```python
from build123d import *

# Parameters (mm, degrees)
CYLINDER068_R     = 71
CYLINDER068_DEPTH = 2
CYLINDER069_R     = 71
CYLINDER069_DEPTH = 2


with BuildPart() as cylinder:
    # Cylinder068 → Cylinder068 (new body)
    with BuildSketch(Plane(origin=(105, 148, 35), x_dir=(1, 0, 0), z_dir=(0, 0, 1))):
        Circle(CYLINDER068_R)
    extrude(amount=CYLINDER068_DEPTH)


with BuildPart() as obj1:
    # Cylinder069 → Cylinder069 (new body)
    with BuildSketch(Plane(origin=(105, 66, 35), x_dir=(1, 0, 0), z_dir=(0, 0, 1))):
        Circle(CYLINDER069_R)
    extrude(amount=CYLINDER069_DEPTH)

    # Common001: intersect Cylinder
    add(cylinder.part, mode=Mode.INTERSECT)


solid = obj1.part
```
Could you check a few things on this model? Use its own coordinates, in mm. Give positions to 0.01 mm unless a question says otherwise; leave off trailing zeros. Order: outer loops, then holes, each group sorted by start corner. A loop starts at its lowest first (then second) coordinate and runs counter-clockwise, first axis right, second up.
Q1. If I drill on line 1 along Y through (x, z) = (106, 35.2); line 2 along X through (y, z) = (108.5, 35.8); line 3 along Y through (x, z) = (87.5, 35.25), over which ranges is the centre line in solid material (lowest first)?
Q2. Suppose I cut it at C-C, the plane y = 101. Write out the boundary of the cut face in (x, z).
Q3. Suppose I cut it at B-B, the plane x = 92.5. Write out the boundary of the cut face in (y, z).
Q4. I'm going to push a flat-ended pin straight in: P1, Ø1, axis at y = 101.5, z = 35.5, coming from the -X side. Where does the tip first touch, or does it pass through?
Q5. Suppose I cut it at A-A, the plane z = 36. Write out the boundary of the cut face in (x, y).
Solution:
1. line 1: y = 77.01 to 136.99
1. line 2: x = 48.13 to 161.87
1. line 3: y = 79.19 to 134.81
2. outline: (51.78, 35) - (158.22, 35) - (158.22, 37) - (51.78, 37) - close
3. outline: (78.11, 35) - (135.89, 35) - (135.89, 37) - (78.11, 37) - close
4. P1: stops at x = 50.92
5. outline: (47.03, 107) arc R71 ccw to (162.97, 107) arc R71 ccw to start
